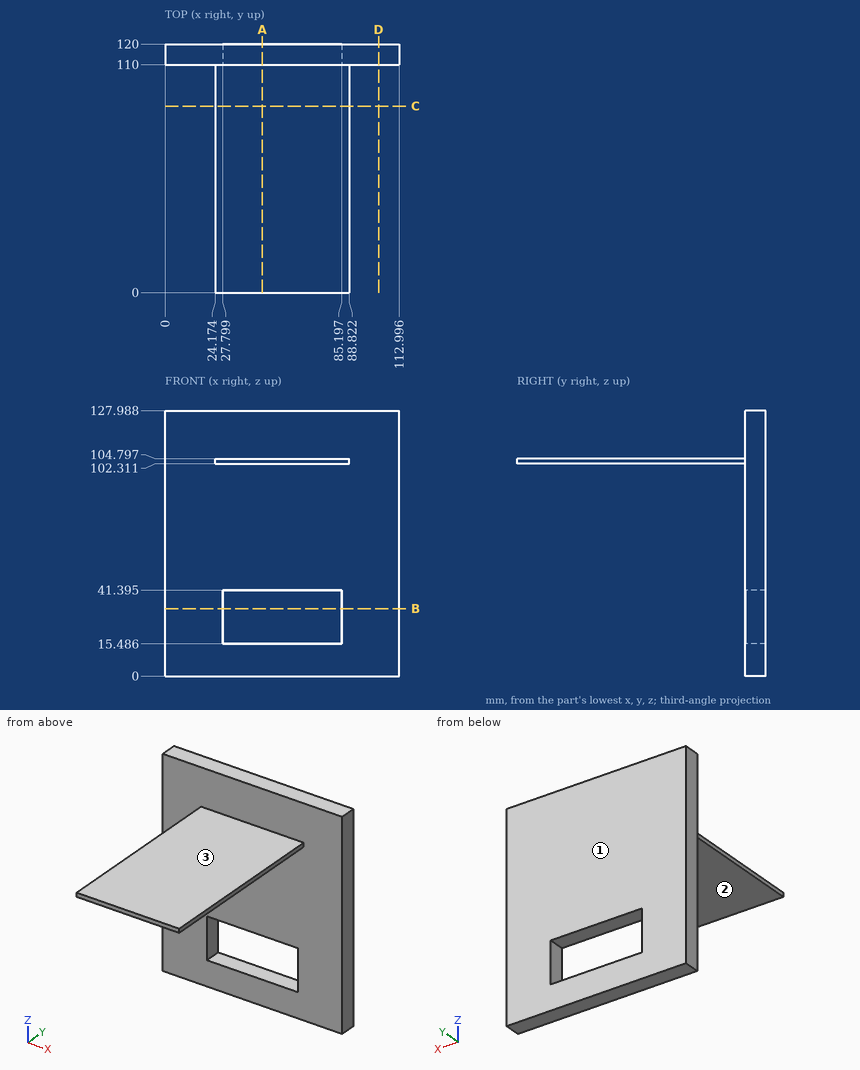
The drawing under review shows one solid part. Ordinate dimensions are in mm from its lowest x, y, z. A direction names the side the tool comes from. Give positions to 0.01 mm unless a question says otherwise; leave off trailing zeros. Order: outer loops, then holes, each group sorted by start corner. A loop starts at its lowest first (then second) coordinate and runs counter-clockwise, first axis right, second up. Notation, with made-up numbers: (59.25, 32) - (95.25, 32) arc R9 cw to (95.25, 48) - close; hole circle Ø2 at (0.5, 43.5). An arc over 180 degrees is marked (long way). Answer as a JSON object with one key per item and string values. Group by question number.
Item 1: Wall thickness on line 1 along Y through (x, z) = (50, 66.5); line 2 along Z through (x, y) = (55, 106): over which ranges is each line inside the solid? List them lowest first.
Item 2: Machinability: for the marked faces 1, 2 and 3, which of the approach directions +Z, -Z, +X, -X, +Y, -Y give a long, thin tool a straight path to every point of the face, cutting with its end or side? Answer none if there is none.
Item 3: Take a section at D-D on x = 103. Give the boundary of the cut face in (y, z), and give its area (3 significant figures).
Item 4: Take a section at C-C on y = 90. Give the boundary of the cut face in (x, z) (1 decimal).
Item 5: Clearance check with flat-ended pins moving along their axes: pin 1 Ø2.5 at (y, z) = (52.5, 103.5) entering from +X; pin 2 Ø3 at (y, z) = (116, 33) entering from -X; pin 3 Ø4 at (x, y) = (30, 75) entering from -Z; pin 4 Ø2.5 at (y, z) = (29.5, 103.5) entering from -X. State where each tip first meets the part, or that it passes through.
Item 6: Take a section at B-B on z = 32.5. Give the boundary of the cut face in (x, y) (1 decimal).
Item 7: Take a section at A-A on x = 47. Give the boundary of the cut face in (y, z) (1 decimal), and give its area (3 significant figures).
Reported:
{
 "1": {"line 1": "110 to 120", "line 2": "102.31 to 104.8"},
 "2": {"face 1": "+Z, -Z, +X, -X, +Y", "face 2": "-Z, +X, -X, -Y", "face 3": "+Z, +X, -X, -Y"},
 "3": {"outline": "(110, 0) - (120, 0) - (120, 127.99) - (110, 127.99) - close", "area": "1,280 mm^2"},
 "4": {"outline": "(24.2, 102.3) - (88.8, 102.3) - (88.8, 104.8) - (24.2, 104.8) - close"},
 "5": {"pin 1": "x = 88.82", "pin 2": "x = 0", "pin 3": "z = 102.31", "pin 4": "x = 24.17"},
 "6": {"outline": "(0, 110) - (27.8, 110) - (27.8, 120) - (0, 120) - close; (85.2, 110) - (113, 110) - (113, 120) - (85.2, 120) - close"},
 "7": {"outline": "(0, 102.3) - (110, 102.3) - (110, 41.4) - (120, 41.4) - (120, 128) - (110, 128) - (110, 104.8) - (0, 104.8) - close; (110, 0) - (120, 0) - (120, 15.5) - (110, 15.5) - close", "area": "1,290 mm^2"}
}
